Design review of the part built by this model. Coordinates are the model's own, in mm. Round coordinates to 2 decimals unless told otherwise and drop trailing zeros. Write each loop counter-clockwise with the first axis right and the second up, starting at its lowest first coordinate (ties: lowest second). Pieces come first, ordered by that corner, then holes. Notation, with made-up numbers: (-35.5, -7.75) -> (-31.5, -7.75) arc R17 cw to (-31.5, 24.25) -> close; hole circle Ø6 at (8, -33). An arc over 180 degrees is marked (long way). Write item = value, one per line. Start each with the question number.
Item 1: To check wall thickness, follow L1, parallel to Y at x = -11.5, z = 0.5; L2, parallel to Y at x = -12.5, z = 0.75; L3, parallel to X at y = 1, z = 1.05. State the ranges of each line that lie inside material, in increasing order.
Item 2: Add section A-A, the plane z = 0.4. State the section outline as (x, y) points, then the cut area to 3 significant figures.
Item 3: For pin 1 Ø0.6 at (x, z) = (1, 0.5) entering from -Y, flat-tipped, find the tip position at first contact; note if it passes through.
Item 4: Add section B-B, the plane x = 13. State how many separate pieces and enclosed holes the cut face has, then the cut area to 3 significant figures.
from build123d import *

# Parameters (mm, degrees)
F0_R     = 17.0734697504
F1_DEPTH = 1.27
F2_SIZE  = 0.508


with BuildPart() as f1:
    # F0 (on Top) → F1 (new body)
    with BuildSketch(Plane.XY):
        Circle(F0_R)
        with BuildLine():
            ThreePointArc((12.0605428134, 9.3167004378), (14.4232498501, 4.9221401608), (15.24, 0))
            ThreePointArc((15.24, 0), (15.2127889804, -0.9103029381), (15.131253092, -1.8173551845))
            ThreePointArc((15.131253092, -1.8173551845), (0, -15.24), (-15.131253092, -1.8173551845))
            ThreePointArc((-15.131253092, -1.8173551845), (-15.2127889804, -0.9103029381), (-15.24, 0))
            ThreePointArc((-15.24, 0), (-14.3893350592, 5.0204219498), (-11.9323049141, 9.4803849835))
            ThreePointArc((-11.9323049141, 9.4803849835), (-11.3577782125, 10.1616176898), (-10.7444158345, 10.8081047541))
            ThreePointArc((-10.7444158345, 10.8081047541), (0, 15.24), (10.7444158345, 10.8081047541))
            ThreePointArc((10.7444158345, 10.8081047541), (11.4268371145, 10.0838977364), (12.0605428134, 9.3167004378))
        make_face(mode=Mode.SUBTRACT)
        with BuildLine():
            Line((-2.5077849958, 0), (0, 0))
            Line((0, 0), (-10.7444158345, 10.8081047541))
            ThreePointArc((-10.7444158345, 10.8081047541), (-11.3577782125, 10.1616176898), (-11.9323049141, 9.4803849835))
            Line((-11.9323049141, 9.4803849835), (-9.5489449564, 7.0828973502))
            Line((-9.5489449564, 7.0828973502), (-2.5077849958, 0))
        make_face()
        with BuildLine():
            Line((2.306102775, 0), (12.0605428134, 9.3167004378))
            ThreePointArc((12.0605428134, 9.3167004378), (11.4268371145, 10.0838977364), (10.7444158345, 10.8081047541))
            Line((10.7444158345, 10.8081047541), (0, 0))
            Line((0, 0), (2.306102775, 0))
        make_face()
        with BuildLine():
            ThreePointArc((15.131253092, -1.8173551845), (15.2127889804, -0.9103029381), (15.24, 0))
            Line((15.24, 0), (2.306102775, 0))
            Line((2.306102775, 0), (0, 0))
            Line((0, 0), (-2.5077849958, 0))
            Line((-2.5077849958, 0), (-15.24, 0))
            ThreePointArc((-15.24, 0), (-15.2127889804, -0.9103029381), (-15.131253092, -1.8173551845))
            Line((-15.131253092, -1.8173551845), (15.131253092, -1.8173551845))
        make_face()
    extrude(amount=F1_DEPTH)

    # F2
    f2_edges = [f1.edges().sort_by_distance(p)[0] for p in [
        (-17.07347, 0, 1.27),
        (0, -15.24, 1.27),
        (-14.389335, 5.020422, 1.27),
        (0, 15.24, 1.27),
        (14.42325, 4.92214, 1.27),
    ]]
    chamfer(f2_edges, length=F2_SIZE)


solid = f1.part
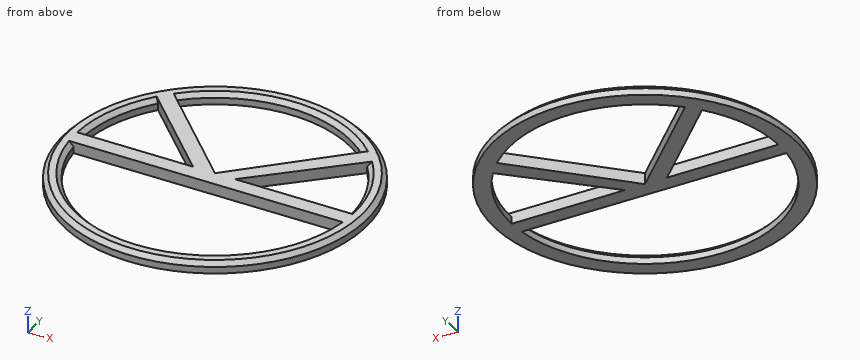
Result set:
q1.L1 = -12.62 to -10, -1.82 to 0, 9.05 to 12.62
q1.L2 = -11.63 to -8.72, -1.82 to 0, 8.72 to 11.63
q1.L3 = -16.76 to -15.5, -3.5 to -0.99, 0.99 to 3.35, 15.5 to 16.76
q2.outline = circle Ø34.15 at (0, 0); hole (-15.24, 0) -> (-2.51, 0) -> (-11.93, 9.48) arc R15.24 ccw to start; hole (-15.13, -1.82) arc R15.24 ccw to (15.13, -1.82) -> close; hole (-10.74, 10.81) -> (0, 0) -> (10.74, 10.81) arc R15.24 ccw to start; hole (2.31, 0) -> (15.24, 0) arc R15.24 ccw to (12.06, 9.32) -> close
q2.area = 293 mm²
q3.pin_1 = -17.06
q4.separate_pieces = 3
q4.enclosed_holes = 0
q4.area = 9.33 mm²
